Geometry: final body of the model. Coordinates: model frame, mm. Face numbers are marked on the shaded views. Give positions to 0.01 mm unless a question says otherwise; leave off trailing zeros. Loops run counter-clockwise (first coordinate to the right, second up) from the corner with the lowest first, then second, coordinate; pieces in that order, holes last. Notation, with made-up numbers: M -17.5,-23 L 34.5,-23 A6 ccw 34.5,-18 Z; hole C 23.5,27.5 d11. An arc over 180 degrees is marked long. Put each result on its own line as item: value.
```python
from build123d import *

# Parameters (mm, degrees)
F1_DEPTH = 3.175


with BuildPart() as f1:
    # F0 (on Top) → F1 (new body)
    with BuildSketch(Plane.XY):
        with BuildLine():
            ThreePointArc((9.525, 0), (0, 9.525), (-9.525, 0))
            ThreePointArc((-9.525, 0), (0, -9.525), (9.525, 0))
        make_face()
        with BuildLine():
            ThreePointArc((-7.9375, 0), (0, 7.9375), (7.9375, 0))
            ThreePointArc((7.9375, 0), (0, -7.9375), (-7.9375, 0))
        make_face(mode=Mode.SUBTRACT)
        with BuildLine():
            Line((-9.525, 11.865028), (-9.525, 0))
            ThreePointArc((-9.525, 0), (0, 9.525), (9.525, 0))
            Line((9.525, 0), (9.525, 11.8618))
            Line((9.525, 11.8618), (6.5532, 11.8618))
            Line((6.5532, 11.8618), (6.5532, 9.8298))
            ThreePointArc((6.5532, 9.8298), (-0.007139, 11.163698), (-6.553978, 9.765045))
            Line((-6.553978, 9.765045), (-6.553978, 11.797045))
            Line((-6.553978, 11.797045), (-9.525, 11.865028))
        make_face()
        with BuildLine():
            ThreePointArc((-6.553978, 11.797045), (-8.00471, 13.350928), (-9.525, 11.865028))
            Line((-9.525, 11.865028), (-6.553978, 11.797045))
        make_face()
        with BuildLine():
            Line((6.5532, 11.8618), (9.525, 11.8618))
            ThreePointArc((9.525, 11.8618), (8.0391, 13.3477), (6.5532, 11.8618))
        make_face()
    extrude(amount=F1_DEPTH)


solid = f1.part
```
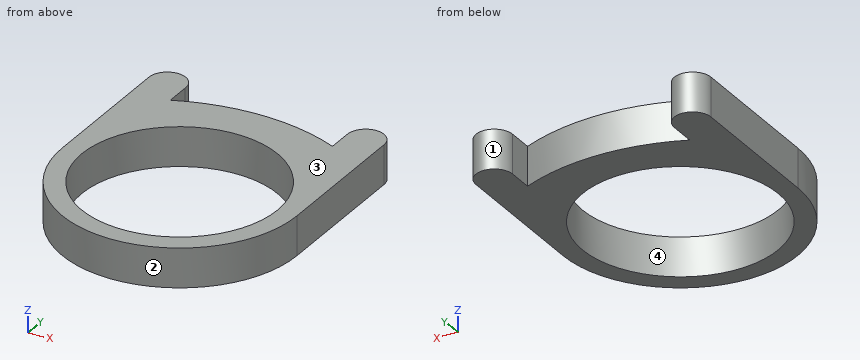
Item 1: Section A-A on x = 0. Output: boundary loops of the cut face in (y, z) (1 decimal), then the cut area to 3 significant figures.
Output values:
outline: M -9.5,0 L -7.9,0 L -7.9,3.2 L -9.5,3.2 Z; M 7.9,0 L 11.2,0 L 11.2,3.2 L 7.9,3.2 Z
area: 15.3 mm²
Item 2: Line query: probe 1 along X at (y, z) = (-0.25, 1.8); probe 2 along Y at (x, z) = (0, 1.05) (1 decimal); probe 3 along Y at (x, z) = (1, 1.95). Output: solid intervals per line, ascending. Write a range as [from, to].
Output values:
probe 1: [-9.52, -7.93], [7.93, 9.52]
probe 2: [-9.5, -7.9], [7.9, 11.2]
probe 3: [-9.47, -7.87], [7.87, 11.14]
Item 3: Pin query (flat end, axial travel): pin 1 Ø1 at (x, z) = (-4, 1) entering from +Y; pin 2 Ø5 at (x, y) = (5.5, -5.5) entering from +Z (3 decimals); pin 3 Ø2 at (x, y) = (-1, -6) entering from -Z. Return the tip coordinate at first contact, or that it passes through.
Output values:
pin 1: y = 10.77
pin 2: z = 3.175
pin 3: through
Item 4: Section B-B on y = -5. Output: boundary loops of the cut face in (x, z) (3 decimals).
Output values:
outline: M -8.107,0 L -6.165,0 L -6.165,3.175 L -8.107,3.175 Z; M 6.165,0 L 8.107,0 L 8.107,3.175 L 6.165,3.175 Z
Item 5: Mould query, pull axis Y, two halves, no side actions, for the marked faces 1, 2, 3 and 4. Classes: pulls with the +Y half, pulls with the -Y half, needs draft (parallel to the pull), parting line crosses it, or undercut.
Output values:
face 1: pulls with the +Y half
face 2: pulls with the -Y half
face 3: needs draft
face 4: undercut
